Job drawing, mm, ordinate dimensions from the low corner. One solid piece. A direction names the side the tool comes from. Coordinates: 2 decimals unless noted, no trailing zeros. Write each loop counter-clockwise with the first axis right and the second up, starting at its lowest first coordinate (ties: lowest second). Pieces come first, ordered by that corner, then holes. Notation, with made-up numbers: (76, 21) - (128, 21) arc R19 ccw to (128, 37) - close; hole circle Ø3 at (84.25, 15.5). An arc over 180 degrees is marked (long way). Use a Markdown table: item, result.
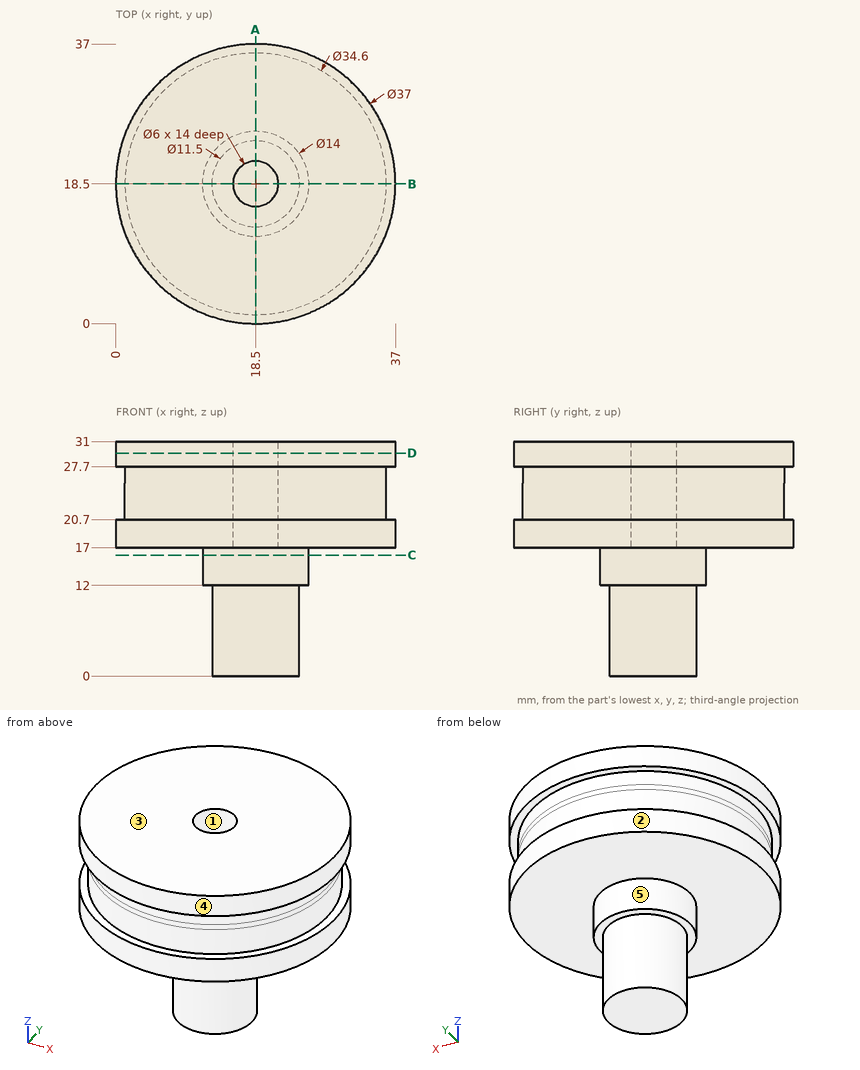
Item 1: Two-plate mould, pull along Y, no slides. Class the marked faces 1, 2 and 3: pulls with the +Y half, pulls with the -Y half, needs draft (parallel to the pull), parting line crosses it, or undercut.
From the geometry:
| item | result |
|---|---|
| face 1 | undercut |
| face 2 | parting line crosses it |
| face 3 | needs draft |
Item 2: Band-saw the part on A-A, the plane x = 18.5. Give the cut face in (y, z).
From the geometry:
| item | result |
|---|---|
| outline | (0, 17) - (11.5, 17) - (11.5, 12) - (12.75, 12) - (12.75, 0) - (24.25, 0) - (24.25, 12) - (25.5, 12) - (25.5, 17) - (37, 17) - (37, 20.7) - (35.8, 20.7) - (35.8, 27.7) - (37, 27.7) - (37, 31) - (21.5, 31) - (21.5, 17) - (15.5, 17) - (15.5, 31) - (0, 31) - (0, 27.7) - (1.2, 27.7) - (1.2, 20.7) - (0, 20.7) - close |
Item 3: Drill centre lines: probe 1 along Y at (x, z) = (18.5, 20); probe 2 along Y at (x, z) = (18.5, 27); probe 3 along Z at (x, y) = (23, 8). Where is each one in solid material? Low to high.
From the geometry:
| item | result |
|---|---|
| probe 1 | 0 to 15.5, 21.5 to 37 |
| probe 2 | 1.2 to 15.5, 21.5 to 35.8 |
| probe 3 | 17 to 31 |
Item 4: Drop flat-ended pins along their axis: P1, Ø6, axis at x = 18, y = 4, coming from the -Z side; P2, Ø10, axis at y = 12.5, z = 24.5, coming from the -X side; P3, Ø11, axis at x = 19, y = 10, coming from the -Z side; P4, Ø8, axis at y = 22.5, z = 11, coming from the -X side. Give the stop position or say it passes through.
From the geometry:
| item | result |
|---|---|
| P1 | z = 17 |
| P2 | x = 0.13 |
| P3 | z = 0 |
| P4 | x = 11.5 |
Item 5: Band-saw the part on D-D, the plane z = 29.5. Give the cut face in (x, y).
From the geometry:
| item | result |
|---|---|
| outline | circle Ø37 at (18.5, 18.5); hole circle Ø6 at (18.5, 18.5) |
Item 6: Band-saw the part on C-C, the plane z = 16. Give the cut face in (x, y).
From the geometry:
| item | result |
|---|---|
| outline | circle Ø14 at (18.5, 18.5) |
Item 7: Which spindle directions (+Z, -Z, +X, -X, +Y, -Y) get a long thin tool onto all of the face, cutting with end or side? Do the marked faces 4 and 5. Say none if no direction does.
From the geometry:
| item | result |
|---|---|
| face 4 | +Z, -Z |
| face 5 | -Z |
